Here's the drawing with two shaded views (mm, measured from the low corner). I have some questions. A direction names the side the tool comes from. Coordinates: 2 decimals unless noted, no trailing zeros. Write each loop counter-clockwise with the first axis right and the second up, starting at its lowest first coordinate (ties: lowest second). Pieces come first, ordered by that corner, then holes.
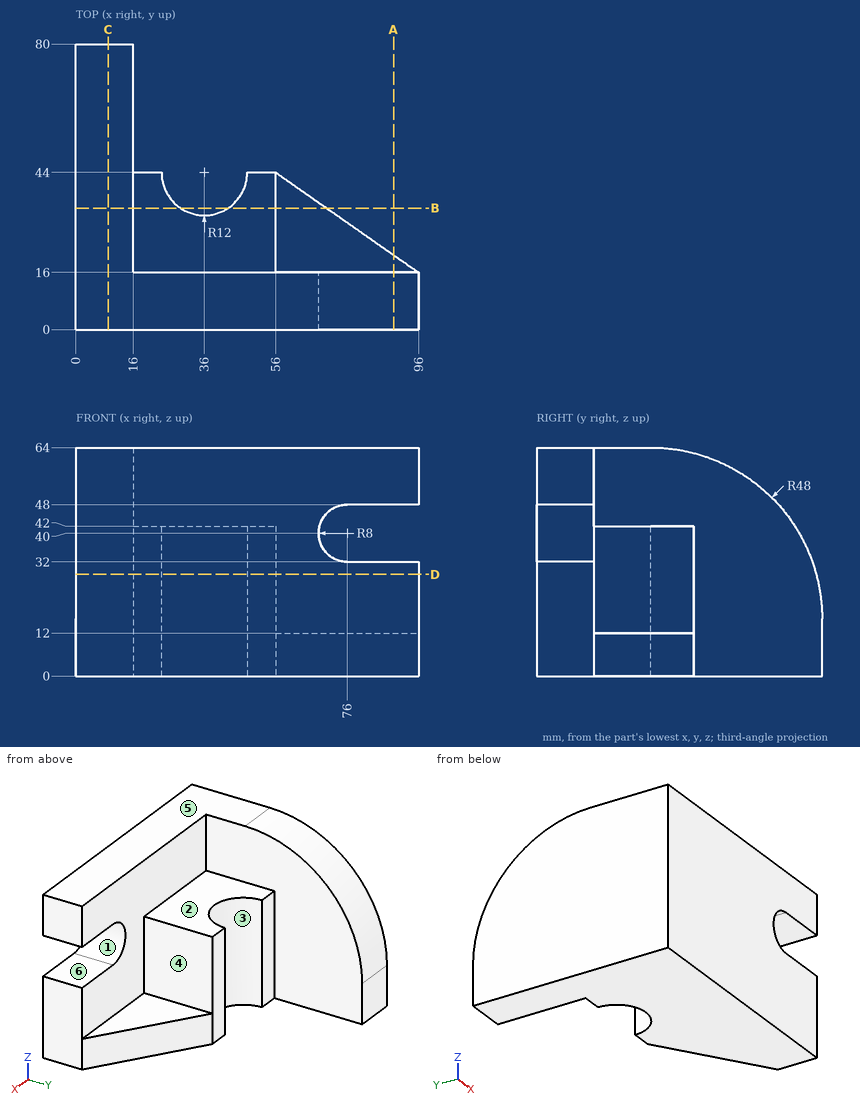
Item 1: Which directions (+Z, -Z, +X, -X, +Y, -Y) give clear straight access to the entire face, cutting with the end or side of a thin tool? Please do the marked faces 4, 5 and 6.
Item 2: I want a section at A-A, the plane x = 89. List the corners of the cut face in (y, z) for me.
Item 3: Will these pins go through, and if not, where does the flat tip stop? pin 1 Ø6.5 at (x, z) = (53, 18.5) entering from +Y; pin 2 Ø8 at (x, z) = (34.5, 48.5) entering from +Y; pin 3 Ø8 at (x, z) = (35.5, 42) entering from +Y.
Item 4: If I drill on line 1 along X through (y, z) = (67, 29); line 2 along X through (y, z) = (40, 32.5), over which ranges is the centre line in solid material (lowest first)?
Item 5: If we mould it in two halves opening along X, with no side actions, what happens to the marked faces 1, 2 and 3? For each: released by +X, released by -X, zero draft, split by the parting line, or undercut.
Item 6: I want a section at B-B, the plane y = 34. List the corners of the cut face in (x, z) for me.
Item 7: I want a section at C-C, the plane x = 9. List the corners of the cut face in (y, z) for me, then the cut area to 3 significant figures.
Item 8: I want a section at D-D, the plane z = 28.5. List the corners of the cut face in (x, y) for me, then the cut area to 3 significant figures.
Taken from the geometry:
1. face 4: +Z, +X, +Y
1. face 5: +Z, +X, -X, +Y, -Y
1. face 6: +X, +Y, -Y
2. outline: (0, 0) - (20.9, 0) - (20.9, 12) - (16, 12) - (16, 32) - (0, 32) - close; (0, 48) - (16, 48) - (16, 64) - (0, 64) - close
3. pin 1: stops at y = 44
3. pin 2: stops at y = 16
3. pin 3: stops at y = 32.88
4. line 1: x = 0 to 16
4. line 2: x = 0 to 24.69, 47.31 to 56
5. face 1: released by +X
5. face 2: zero draft
5. face 3: undercut
6. outline: (0, 0) - (29.37, 0) - (29.37, 42) - (16, 42) - (16, 63.96) - (0, 63.96) - close; (42.63, 0) - (70.29, 0) - (70.29, 12) - (56, 12) - (56, 42) - (42.63, 42) - close
7. outline: (0, 0) - (80, 0) - (80, 16) arc R48 ccw to (32, 64) - (0, 64) - close
7. area: 4,630 mm2
8. outline: (0, 0) - (96, 0) - (96, 16) - (56, 16) - (56, 44) - (48, 44) arc R12 cw to (24, 44) - (16, 44) - (16, 78.34) - (0, 78.34) - close
8. area: 3,430 mm2
